Source: CAD feature listing. Evaluate the final solid. Frame: model axes, mm. Round coordinates to 2 decimals unless told otherwise and drop trailing zeros. Loops run counter-clockwise (first coordinate to the right, second up) from the corner with the lowest first, then second, coordinate; pieces in that order, holes last. Notation, with made-up numbers: (-10, 19) -> (3, 19) arc R29 ccw to (3, 51) -> close; hole circle Ø11 at (10.5, -22.5). An arc over 180 degrees is marked (long way). Return JSON: item names as keys, results as strings. Group by question number.
```python
from build123d import *

# Parameters (mm, degrees)
BOSS_EXTRUDE3_DEPTH      = 34
BOSS_EXTRUDE3_DEPTH_BACK = 34
SKETCH1_R                = 4.7625
CUT_EXTRUDE1_DEPTH       = 36.469734281
CUT_EXTRUDE3_DEPTH       = 36.46973442
CUT_EXTRUDE3_DEPTH_BACK  = 36.46973442


with BuildPart() as part:
    # Sketch2 → Boss-Extrude3 (new, two sides)
    with BuildSketch(Plane(origin=(0, 0, 0), x_dir=(0, 0, -1), z_dir=(1, 0, 0))) as boss_extrude3_sk:
        with BuildLine():
            Line((-7.145, 0), (7.145, 0))
            ThreePointArc((7.145, 0), (0, -7.145), (-7.145, 0))
        make_face()
    extrude(amount=BOSS_EXTRUDE3_DEPTH)
    extrude(boss_extrude3_sk.sketch, amount=-BOSS_EXTRUDE3_DEPTH_BACK)

    # Sketch1 → Cut-Extrude1 (cut, through all)
    with BuildSketch(Plane(origin=(0, 0, 0), x_dir=(1, 0, 0), z_dir=(0, 1, 0))):
        with Locations(Location((-20, 0, 0), (0, 0, 270))):
            Circle(SKETCH1_R)
        with Locations((20, 0)):
            Circle(SKETCH1_R)
    extrude(amount=-CUT_EXTRUDE1_DEPTH, mode=Mode.SUBTRACT)

    # Sketch4 → Cut-Extrude3 (cut, two sides)
    with BuildSketch(Plane.XY) as cut_extrude3_sk:
        Polygon((-13, 0), (13, 0), (7.803847577, -9), (-7.803847577, -9), align=None)
        Polygon((32.196152423, -9), (43.216463998, -9), (43.216463998, 0), (27, 0), align=None)
        Polygon((-43.216463998, 0), (-27, 0), (-32.196152423, -9), (-43.216463998, -9), align=None)
    extrude(amount=CUT_EXTRUDE3_DEPTH, mode=Mode.SUBTRACT)
    extrude(cut_extrude3_sk.sketch, amount=-CUT_EXTRUDE3_DEPTH_BACK, mode=Mode.SUBTRACT)


with BuildPart() as cut_extrude3_piece_1:
    # of the separate pieces the step leaves, piece 1, a body of its own (cut_extrude3_pieces)
    add(part.part.solids().sort_by_distance((-27, 0, 7.145))[0])


with BuildPart() as cut_extrude3_piece_2:
    # of the separate pieces the step leaves, piece 2, a body of its own (cut_extrude3_pieces)
    add(part.part.solids().sort_by_distance((13, 0, 7.145))[0])


solid = cut_extrude3_piece_2.part
```
(1) Cut plane D-D (y = -2.75). Return loops of the section in (x, z) (1 decimal), and give its area (3 significant figures).
(2) Pin query (flat end, axial travel): pin 1 (1 mm diameter, centred on x = 18.5, y = -4, fed in from +Z); pin 2 (5 mm diameter, centred on x = 24, z = -0.5, fed in from -Y) (3 decimals); pin 3 (7.5 mm diameter, centred on x = 20, z = 0, fed in from +Y). Return the tip coordinate at first contact, or that it passes through.
(3) Mould query, pull axis X, two halves, no side actions, for faces 1 (the face through (24.4, -2.73, 1.82)), 2 (the face through (28.575, -2.729, -0.1)), 3 (the face through (22.628, -5.573, 4.471)), 4 (the face through (11.425, -2.729, -0.1)). Classes: released by +X, released by -X, zero draft, split by the parting line, or undercut.
(4) Cut plane B-B (x = 20). Return loops of the section in (y, z) (1 decimal), and give its area (3 significant figures).
(5) Cut plane A-A (z = 0). Return loops of the section in (x, y) (1 decimal).
(6) Ray query, line 1 (X direction, y = -5.5, z = -3); line 2 (X direction, y = -4.75, z = 0.5); line 3 (Z direction, x = 18.5, y = -0.5). Return the intervals inside material, ascending.
(7) Cut plane C-C (y = -5.5). Return loops of the section in (x, z) (1 decimal).
Answers follow:
{
 "1": {"outline": "(11.4, -6.6) -> (28.6, -6.6) -> (28.6, 6.6) -> (11.4, 6.6) -> close; hole circle Ø9.5 at (20, 0)", "area": "155 mm^2"},
 "2": {"pin 1": "z = 6.23", "pin 2": "y = -7.145", "pin 3": "through"},
 "3": {"face 1": "undercut", "face 2": "released by +X", "face 3": "zero draft", "face 4": "released by -X"},
 "4": {"outline": "(-5.3, -4.8) arc R7.1 ccw to (0, -7.1) -> (0, -4.8) -> close; (-5.3, 4.8) -> (0, 4.8) -> (0, 7.1) arc R7.1 ccw to start", "area": "17.6 mm^2"},
 "5": {"outline": "(8.9, -7.1) -> (15.2, -7.1) -> (15.2, 0) -> (13, 0) -> close; (24.8, -7.1) -> (31.1, -7.1) -> (27, 0) -> (24.8, 0) -> close"},
 "6": {"line 1": "9.82 to 16.3, 23.7 to 30.18", "line 2": "10.26 to 15.26, 24.74 to 29.74", "line 3": "-7.13 to -4.52, 4.52 to 7.13"},
 "7": {"outline": "(9.8, -4.6) -> (18.6, -4.6) arc R4.8 cw to (18.6, 4.6) -> (9.8, 4.6) -> close; (21.4, -4.6) -> (30.2, -4.6) -> (30.2, 4.6) -> (21.4, 4.6) arc R4.8 cw to start"}
}
